Source: CAD feature listing. Evaluate the final solid. Frame: model axes, mm. A direction names the side the tool comes from. Give positions to 0.01 mm unless a question says otherwise; leave off trailing zeros. Write each loop counter-clockwise with the first axis right and the second up, starting at its lowest first coordinate (ties: lowest second). Pieces come first, ordered by that corner, then holes. Notation, with made-up numbers: (50, -24.75) -> (101, -24.75) arc R31 cw to (101, 9.25) -> close; hole circle Ø1 at (-18.5, 5.5). An arc over 180 degrees is marked (long way). Write item = value, one per line.
from build123d import *

# Parameters (mm, degrees)
F0_R     = 7.25
F0_R_2   = 2.5
F1_DEPTH = 5
F2_R     = 3.5
F2_R_2   = 2.5
F3_DEPTH = 3
F4_R     = 1


with BuildPart() as f1:
    # F0 (on Top) → F1 (new body)
    with BuildSketch(Plane.XY):
        Circle(F0_R)
        Circle(F0_R_2, mode=Mode.SUBTRACT)
    extrude(amount=F1_DEPTH)

    # F2 (on face) → F3 (cut)
    with BuildSketch(Plane.XY.offset(5)):
        Circle(F2_R)
        Circle(F2_R_2, mode=Mode.SUBTRACT)
    extrude(amount=-F3_DEPTH, mode=Mode.SUBTRACT)

    # F4
    f4_edges = [f1.edges().sort_by_distance(p)[0] for p in [
        (-7.25, 0, 5),
        (-3.5, 0, 5),
        (-7.25, 0, 0),
    ]]
    fillet(f4_edges, radius=F4_R)


solid = f1.part
(1) Section query A-A (y = 0). Return loops of the section in (x, z), plus the area to 3 significant figures.
Values follow:
outline = (-7.25, 1) arc R1 ccw to (-6.25, 0) -> (-2.5, 0) -> (-2.5, 2) -> (-3.5, 2) -> (-3.5, 4) arc R1 ccw to (-4.5, 5) -> (-6.25, 5) arc R1 ccw to (-7.25, 4) -> close; (2.5, 0) -> (6.25, 0) arc R1 ccw to (7.25, 1) -> (7.25, 4) arc R1 ccw to (6.25, 5) -> (4.5, 5) arc R1 ccw to (3.5, 4) -> (3.5, 2) -> (2.5, 2) -> close
area = 40.2 mm2
(2) First-contact query: pin 1 (5 mm diameter, centred on x = 5.5, y = 2.5, fed in from -Z); pin 2 (2 mm diameter, centred on x = -5.5, z = 4, fed in from +Y); pin 3 (1.5 mm diameter, centred on y = 1.5, z = 1.5, fed in from +X); pin 4 (5.5 mm diameter, centred on x = 1.5, y = -0.5, fed in from +Z). Flat tips, straight axial feed; report the tip coordinate or a pass-through.
Values follow:
pin_1 = 0
pin_2 = 5.68
pin_3 = 7.21
pin_4 = 4.99
(3) Access query for faces 1 (the face through (3.233, -1.341, 3.014)), 2 (the face through (0, -3, 0)). Directions: +Z, -Z, +X, -X, +Y, -Y. A direction counts if a zero-diameter tool reaches every point of the face in a straight line with its end or side. Return the directions, or none.
Values follow:
face_1 = +Z
face_2 = -Z, +X, -X, +Y, -Y
(4) Material intervals for line 1 (Y direction, x = 0, z = 2.5); line 2 (Y direction, x = 0, z = 1.5); line 3 (Z direction, x = 0.5, y = -2.75), sorted ascending.
Values follow:
line_1 = -7.25 to -3.5, 3.5 to 7.25
line_2 = -7.25 to -2.5, 2.5 to 7.25
line_3 = 0 to 2
(5) Section query C-C (z = 2.5). Return loops of the section in (x, y), plus the area to 3 significant figures.
Values follow:
outline = circle Ø14.5 at (0, 0); hole circle Ø7 at (0, 0)
area = 127 mm2
